from build123d import *

# Parameters (mm, degrees)
SKETCH1_W           = 26
SKETCH1_H           = 15
BOSS_EXTRUDE1_DEPTH = 17.4
SKETCH3_W           = 23
SKETCH3_H           = 12
CUT_EXTRUDE1_DEPTH  = 15.9
SKETCH5_W           = 12
SKETCH5_H           = 12.9
CUT_EXTRUDE2_DEPTH  = 15.9
SKETCH8_W           = 12.9
SKETCH8_H           = 4.8
CUT_EXTRUDE4_DEPTH  = 1000
SKETCH9_W           = 16
SKETCH9_H           = 6.8
CUT_EXTRUDE5_DEPTH  = 1000
SKETCH10_W          = 1.9
SKETCH10_H          = 15
CUT_EXTRUDE6_DEPTH  = 1000
SKETCH11_R          = 2.175
BOSS_EXTRUDE2_DEPTH = 7.76
BOSS_EXTRUDE3_START = 7.76
SKETCH12_R          = 2.175
SKETCH12_R_2        = 2.18
BOSS_EXTRUDE3_DEPTH = 7.76
SKETCH13_W          = 12
SKETCH13_H          = 11
BOSS_EXTRUDE5_DEPTH = 1.5
SKETCH14_W          = 12
SKETCH14_H          = 11
BOSS_EXTRUDE6_DEPTH = 1.5
SKETCH17_W          = 7.294957973
SKETCH17_H          = 11
CUT_EXTRUDE7_DEPTH  = 50


with BuildPart() as part:
    # Sketch1 → Boss-Extrude1 (new body)
    with BuildSketch(Plane.XY):
        with Locations((13, 7.5)):
            Rectangle(SKETCH1_W, SKETCH1_H)
    extrude(amount=BOSS_EXTRUDE1_DEPTH)

    # Sketch3 → Cut-Extrude1 (cut)
    with BuildSketch(Plane.XY.offset(17.4)):
        with Locations((13, 7.5)):
            Rectangle(SKETCH3_W, SKETCH3_H)
    extrude(amount=-CUT_EXTRUDE1_DEPTH, mode=Mode.SUBTRACT)

    # Sketch5 → Cut-Extrude2 (cut)
    with BuildSketch(Plane.XZ):
        with Locations((13, 10.95)):
            Rectangle(SKETCH5_W, SKETCH5_H)
    extrude(amount=-CUT_EXTRUDE2_DEPTH, mode=Mode.SUBTRACT)

    # Sketch8 → Cut-Extrude4 (cut)
    with BuildSketch(Plane.ZY):
        with Locations((10.95, 7.4)):
            Rectangle(SKETCH8_W, SKETCH8_H)
    extrude(amount=-CUT_EXTRUDE4_DEPTH, mode=Mode.SUBTRACT)

    # Sketch9 → Cut-Extrude5 (cut)
    with BuildSketch(Plane(origin=(0, 0, 0), x_dir=(-1, 0, 0), z_dir=(0, 0, -1))):
        with Locations((-13, 7.4)):
            Rectangle(SKETCH9_W, SKETCH9_H)
    extrude(amount=-CUT_EXTRUDE5_DEPTH, mode=Mode.SUBTRACT)

    # Sketch10 → Cut-Extrude6 (cut)
    with BuildSketch(Plane.ZY):
        with Locations((16.45, 7.5)):
            Rectangle(SKETCH10_W, SKETCH10_H)
    extrude(amount=-CUT_EXTRUDE6_DEPTH, mode=Mode.SUBTRACT)

    # Sketch11 → Boss-Extrude2 (add)
    with BuildSketch(Plane(origin=(0, 15, 0), x_dir=(1, 0, 0), z_dir=(0, 1, 0))):
        with Locations(Location((20.52, -5.805, 0), (0, 0, 143.130102354))):
            Circle(SKETCH11_R)
        with Locations(Location((20.52, -13.32, 0), (0, 0, 134.33485804))):
            Circle(SKETCH11_R)
        with Locations(Location((5.48, -5.805, 0), (0, 0, 90))):
            Circle(SKETCH11_R)
        with Locations(Location((5.48, -13.32, 0), (0, 0, 90))):
            Circle(SKETCH11_R)
    extrude(amount=BOSS_EXTRUDE2_DEPTH)

    # Sketch12 → Boss-Extrude3 (add)
    with BuildSketch(Plane(origin=(0, 0, 0), x_dir=(-1, 0, 0), z_dir=(0, -1, 0)).offset(BOSS_EXTRUDE3_START)):
        with Locations(Location((-5.48, -5.805, 0), (0, 0, 90))):
            Circle(SKETCH12_R)
        with Locations(Location((-5.48, -13.32, 0), (0, 0, 270))):
            Circle(SKETCH12_R_2)
        with Locations(Location((-20.52, -5.805, 0), (0, 0, 36.869897646))):
            Circle(SKETCH12_R)
        with Locations(Location((-20.52, -13.32, 0), (0, 0, 270))):
            Circle(SKETCH12_R_2)
    extrude(amount=-BOSS_EXTRUDE3_DEPTH)

    # Sketch13 → Boss-Extrude5 (add)
    with BuildSketch(Plane(origin=(0, 15, 0), x_dir=(1, 0, 0), z_dir=(0, 1, 0))):
        with Locations((13, -10)):
            Rectangle(SKETCH13_W, SKETCH13_H)
    extrude(amount=-BOSS_EXTRUDE5_DEPTH)

    # Sketch14 → Boss-Extrude6 (add)
    with BuildSketch(Plane(origin=(0, 0, 0), x_dir=(-1, 0, 0), z_dir=(0, -1, 0))):
        with Locations((-13, -10)):
            Rectangle(SKETCH14_W, SKETCH14_H)
    extrude(amount=-BOSS_EXTRUDE6_DEPTH)

    # Sketch17 → Cut-Extrude7 (cut)
    with BuildSketch(Plane(origin=(0, 15, 0), x_dir=(1, 0, 0), z_dir=(0, 1, 0))):
        with Locations((13.002478986, -10)):
            Rectangle(SKETCH17_W, SKETCH17_H)
    extrude(amount=-CUT_EXTRUDE7_DEPTH, mode=Mode.SUBTRACT)


solid = part.part
For this review, take the finished solid that the model builds, in its own axes (mm). A direction names the side the tool comes from. Round coordinates to 2 decimals unless told otherwise and drop trailing zeros. Order: outer loops, then holes, each group sorted by start corner. A loop starts at its lowest first (then second) coordinate and runs counter-clockwise, first axis right, second up. Notation, with made-up numbers: (-24, -30) -> (0, -30) arc R24 ccw to (0, -7) -> close; hole circle Ø7 at (20, 65.5). An arc over 180 degrees is marked (long way). Write item = value, one per line. Start each with the question number.
1) The part is to be moulded in two halves that separate along Z. For faces 1 (the face through (7.314, -3.934, 4.636)), 2 (the face through (22.695, 18.826, 5.782)), 3 (the face through (4, 14, 15.5)), 4 (the face through (21, 7, 1)), say which applies: +Z half, -Z half, draft (parallel to the pull), parting line (faces both ways), or undercut.
2) Take a section at B-B on z = 9. State the section outline as (x, y) points (3 decimals), plus the area to 3 significant figures.
3) To check wall thickness, follow line 1 (Y direction, x = 7.25, z = 15); line 2 (Y direction, x = 7.75, z = 1); line 3 (X direction, y = 14.5, z = 12.5) (3 decimals). State the ranges of each line that lie inside material, in increasing order. Write a range as from..to.
4) Take a section at A-A on x = 17.75. State the section outline as (y, z) points, plus the area to 3 significant figures.
5) Take a section at D-D on x = 2.25. State the section outline as (y, z) points.
6) Tool access review of faces 5 (the face through (13, 12, 1.5)), 6 (the face through (9.355, 14, 10)), 7 (the face through (25, 5, 10)), 8 (the face through (13, 15, 4)): name each direction out of +Z, -Z, +X, -X, +Y, -Y from which nothing blocks a thin tool from reaching the whole face with its end or side.
7) Take a section at C-C on y = 3. State the section outline as (x, z) points.
8) Insertion check: pin 1 (1.2 mm diameter, centred on x = 0.5, z = 8.5, fed in from -Y); pin 2 (5 mm diameter, centred on x = 18, y = 5, fed in from +Z); pin 3 (5 mm diameter, centred on y = 18.5, z = 5, fed in from -X) (3 decimals); pin 4 (3.5 mm diameter, centred on y = 7.5, z = 9, fed in from +X). Each pin has a flat end and moves straight along its axis. Give the tip position at first contact, or say it passes through.
Verdict:
q1.face_1 = undercut
q1.face_2 = undercut
q1.face_3 = +Z half
q1.face_4 = draft
q2.outline = (0, 0) -> (9.355, 0) -> (9.355, 1.5) -> (1.5, 1.5) -> (1.5, 5) -> (0, 5) -> close; (0, 9.8) -> (1.5, 9.8) -> (1.5, 13.5) -> (9.355, 13.5) -> (9.355, 15) -> (0, 15) -> close; (16.65, 0) -> (26, 0) -> (26, 5) -> (24.5, 5) -> (24.5, 1.5) -> (16.65, 1.5) -> close; (16.65, 13.5) -> (24.5, 13.5) -> (24.5, 9.8) -> (26, 9.8) -> (26, 15) -> (16.65, 15) -> close
q2.area = 77.7 mm2
q3.line_1 = 0..1.5, 13.5..15
q3.line_2 = 0..4, 10.8..15
q3.line_3 = 0..9.355, 16.65..26
q4.outline = (0, 0) -> (4, 0) -> (4, 1.5) -> (1.5, 1.5) -> (1.5, 15.5) -> (0, 15.5) -> close; (10.8, 0) -> (15, 0) -> (15, 15.5) -> (13.5, 15.5) -> (13.5, 1.5) -> (10.8, 1.5) -> close
q4.area = 54.3 mm2
q5.outline = (0, 0) -> (15, 0) -> (15, 15.5) -> (13.5, 15.5) -> (13.5, 1.5) -> (1.5, 1.5) -> (1.5, 15.5) -> (0, 15.5) -> close
q6.face_5 = +Z
q6.face_6 = +Z, +Y, -Y
q6.face_7 = +Z, +X, -X
q6.face_8 = +Y
q7.outline = (0, 0) -> (26, 0) -> (26, 15.5) -> (24.5, 15.5) -> (24.5, 1.5) -> (1.5, 1.5) -> (1.5, 15.5) -> (0, 15.5) -> close
q8.pin_1 = 0
q8.pin_2 = 1.5
q8.pin_3 = 3.305
q8.pin_4 = through
